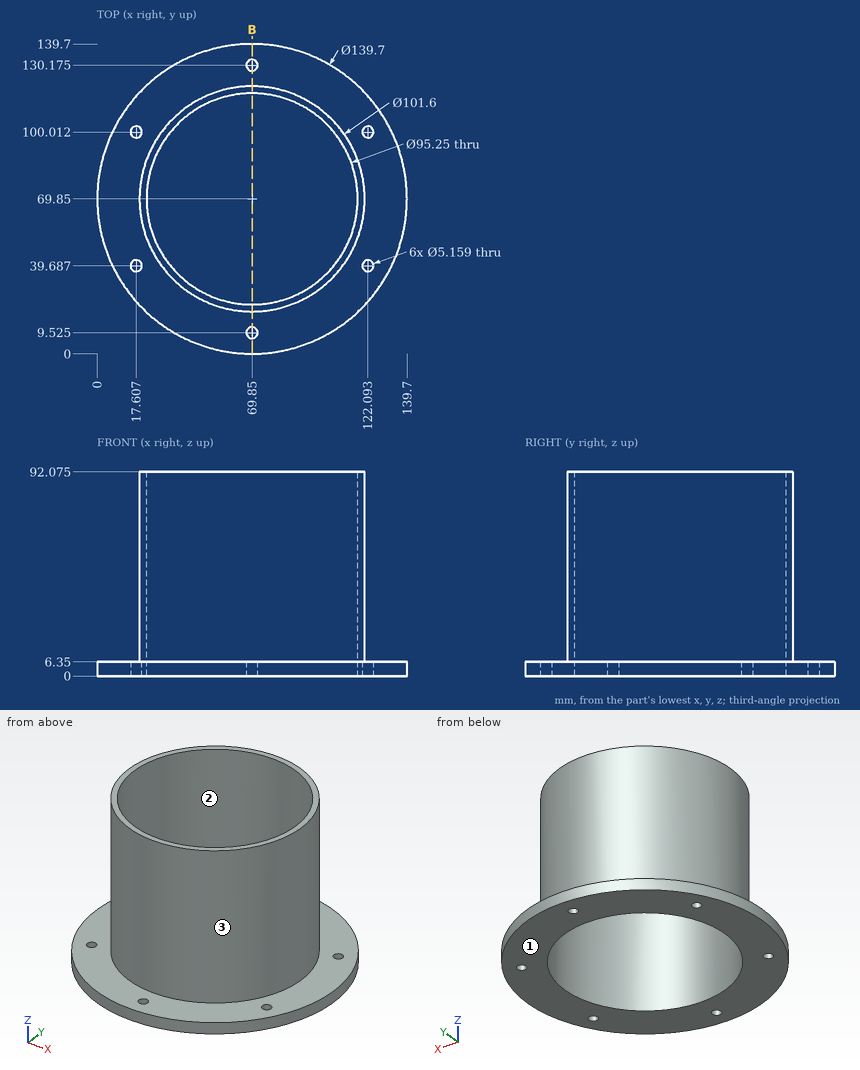
Input: dimensioned drawing with shaded views. Units: mm. Origin: part minimum x, y, z. Round coordinates to 2 decimals unless told otherwise and drop trailing zeros.
Q1. Mould query, pull axis Y, two halves, no side actions, for the marked faces 1, 2 and 3. Classes: released by +Y, released by -Y, zero draft, split by the parting line, or undercut.
Result sheet:
face 1: zero draft
face 2: undercut
face 3: split by the parting line
Q2. Material intervals for probe 1 along Y at (x, z) = (69.85, 1.75) (1 decimal); probe 2 along X at (y, z) = (30, 41.5) (1 decimal); probe 3 along Y at (x, z) = (70.5, 20) (1 decimal), sorted ascending.
Result sheet:
probe 1: y = 0 to 6.9, 12.1 to 22.2, 117.5 to 127.6, 132.8 to 139.7
probe 2: x = 38.3 to 43.8, 95.9 to 101.4
probe 3: y = 19.1 to 22.2, 117.5 to 120.6
Q3. Pin query (flat end, axial travel): pin 1 (3 mm diameter, centred on x = 17.61, y = 100.01, fed in from +Z); pin 2 (2 mm diameter, centred on x = 24.5, z = 78.5, fed in from +Y) (1 decimal); pin 3 (12 mm diameter, centred on y = 117.5, z = 41.5, fed in from +X) (1 decimal); pin 4 (5 mm diameter, centred on x = 53.5, z = 44.5, fed in from +Y) (1 decimal). Return the tip coordinate at first contact, or that it passes through.
Result sheet:
pin 1: passes through
pin 2: stops at y = 94.6
pin 3: stops at x = 98.9
pin 4: stops at y = 118.7
Q4. Section B-B, the plane x = 69.85. Give the number of separate pieces and of enclosed holes in the cut face.
Result sheet:
separate pieces: 4
enclosed holes: 0
